Can you work these out from the model? Positions are in its coordinate system, mm. Round coordinates to 2 decimals unless told otherwise and drop trailing zeros. Loops run counter-clockwise (first coordinate to the right, second up) from the corner with the lowest first, then second, coordinate; pieces in that order, holes last.
from build123d import *

# Parameters (mm, degrees)
SKETCH_1_W               = 10.16
SKETCH_1_H               = 5.08
EXTRUDE_1_DEPTH          = 8
SKETCH_2_W               = 0.6
SKETCH_2_H               = 0.6
CUT_EXTRUDE_1_DEPTH      = 10.811116144
CHAMFER_1_SIZE           = 0.5
CHAMFER_2_SIZE           = 0.5
FILLET_1_R               = 0.05
SKETCH_4_W               = 0.6
SKETCH_4_H               = 0.25
EXTRUDE_3_DEPTH          = 1
PATTERN_LINEAR_2_COUNT   = 4
PATTERN_LINEAR_2_PITCH   = 2.54
MIRROR_1_COPY_1_SKETCH_W = 0.6
MIRROR_1_COPY_1_SKETCH_H = 0.25
MIRROR_1_COPY_1_DEPTH    = 1
MIRROR_1_COPY_2_SKETCH_W = 0.6
MIRROR_1_COPY_2_SKETCH_H = 0.25
MIRROR_1_COPY_2_DEPTH    = 1
MIRROR_1_COPY_3_SKETCH_W = 0.6
MIRROR_1_COPY_3_SKETCH_H = 0.25
MIRROR_1_COPY_3_DEPTH    = 1


with BuildPart() as part:
    # 草图1 → 凸台-拉伸1 (new body)
    with BuildSketch(Plane.XY):
        Rectangle(SKETCH_1_W, SKETCH_1_H)
    extrude(amount=EXTRUDE_1_DEPTH)

    # 草图2 → 切除-拉伸1 (cut, through all)
    with BuildSketch(Plane.XY.offset(8)):
        with Locations((1.27, 1.27)):
            Rectangle(SKETCH_2_W, SKETCH_2_H)
        with Locations((-1.27, 1.27)):
            Rectangle(SKETCH_2_W, SKETCH_2_H)
        with Locations((3.81, 1.27)):
            Rectangle(SKETCH_2_W, SKETCH_2_H)
        with Locations((-1.27, -1.27)):
            Rectangle(SKETCH_2_W, SKETCH_2_H)
        with Locations((1.27, -1.27)):
            Rectangle(SKETCH_2_W, SKETCH_2_H)
        with Locations((3.81, -1.27)):
            Rectangle(SKETCH_2_W, SKETCH_2_H)
        with Locations((-3.81, -1.27)):
            Rectangle(SKETCH_2_W, SKETCH_2_H)
        with Locations((-3.81, 1.27)):
            Rectangle(SKETCH_2_W, SKETCH_2_H)
    extrude(amount=-CUT_EXTRUDE_1_DEPTH, mode=Mode.SUBTRACT)

    # 倒角1
    chamfer_1_edges = [part.edges().sort_by_distance(p)[0] for p in [
        (-3.81, 1.57, 0),
        (-3.51, 1.27, 0),
        (-3.81, 0.97, 0),
        (-4.11, 1.27, 0),
        (-0.97, 1.27, 0),
        (-1.27, 0.97, 0),
        (-1.57, 1.27, 0),
        (-1.27, 1.57, 0),
        (1.57, 1.27, 0),
        (1.27, 0.97, 0),
        (0.97, 1.27, 0),
        (1.27, 1.57, 0),
        (-3.81, -0.97, 0),
        (-3.51, -1.27, 0),
        (-3.81, -1.57, 0),
        (-4.11, -1.27, 0),
        (4.11, 1.27, 0),
        (3.81, 0.97, 0),
        (3.51, 1.27, 0),
        (3.81, 1.57, 0),
        (-0.97, -1.27, 0),
        (-1.27, -1.57, 0),
        (-1.57, -1.27, 0),
        (-1.27, -0.97, 0),
        (1.57, -1.27, 0),
        (1.27, -1.57, 0),
        (0.97, -1.27, 0),
        (1.27, -0.97, 0),
        (4.11, -1.27, 0),
        (3.81, -1.57, 0),
        (3.51, -1.27, 0),
        (3.81, -0.97, 0),
        (4.11, -1.27, 8),
        (3.81, -0.97, 8),
        (3.51, -1.27, 8),
        (3.81, -1.57, 8),
    ]]
    chamfer(chamfer_1_edges, length=CHAMFER_1_SIZE)

    # 倒角2
    chamfer_2_edges = [part.edges().sort_by_distance(p)[0] for p in [
        (-3.81, 1.57, 8),
        (-4.11, 1.27, 8),
        (-3.81, 0.97, 8),
        (-3.51, 1.27, 8),
        (-0.97, 1.27, 8),
        (-1.27, 1.57, 8),
        (-1.57, 1.27, 8),
        (-1.27, 0.97, 8),
        (1.57, 1.27, 8),
        (1.27, 1.57, 8),
        (0.97, 1.27, 8),
        (1.27, 0.97, 8),
        (-3.81, -0.97, 8),
        (-4.11, -1.27, 8),
        (-3.81, -1.57, 8),
        (-3.51, -1.27, 8),
        (4.11, 1.27, 8),
        (3.81, 1.57, 8),
        (3.51, 1.27, 8),
        (3.81, 0.97, 8),
        (-0.97, -1.27, 8),
        (-1.27, -0.97, 8),
        (-1.57, -1.27, 8),
        (-1.27, -1.57, 8),
        (1.57, -1.27, 8),
        (1.27, -0.97, 8),
        (0.97, -1.27, 8),
        (1.27, -1.57, 8),
    ]]
    chamfer(chamfer_2_edges, length=CHAMFER_2_SIZE)

    # 圆角1
    fillet_1_edges = [part.edges().sort_by_distance(p)[0] for p in [
        (-5.08, 0, 8),
        (0, -2.54, 8),
        (5.08, 0, 8),
        (0, 2.54, 8),
        (5.08, -2.54, 4),
        (-5.08, -2.54, 4),
        (-5.08, 2.54, 4),
        (5.08, 2.54, 4),
    ]]
    fillet(fillet_1_edges, radius=FILLET_1_R)

    # 草图4 → 凸台-拉伸3 (add)
    with BuildSketch(Plane(origin=(0, 2.54, 0), x_dir=(1, 0, 0), z_dir=(0, 1, 0))):
        with Locations((-3.81, -0.125)):
            Rectangle(SKETCH_4_W, SKETCH_4_H)
    extrude_3 = extrude(amount=EXTRUDE_3_DEPTH)

    # 阵列(线性)2: 凸台-拉伸3 ×4
    with Locations(*[(i * PATTERN_LINEAR_2_PITCH, 0, 0) for i in range(1, PATTERN_LINEAR_2_COUNT)]):
        add(extrude_3)

    # 镜向1: 凸台-拉伸3 across plane
    add(extrude_3.mirror(Plane.ZX))

    # 镜向1 copy 1 sketch → 镜向1 copy 1 (add)
    with BuildSketch(Plane(origin=(2.54, -2.54, 0), x_dir=(1, 0, 0), z_dir=(0, -1, 0))):
        with Locations((-3.81, 0.125)):
            Rectangle(MIRROR_1_COPY_1_SKETCH_W, MIRROR_1_COPY_1_SKETCH_H)
    extrude(amount=MIRROR_1_COPY_1_DEPTH)

    # 镜向1 copy 2 sketch → 镜向1 copy 2 (add)
    with BuildSketch(Plane(origin=(5.08, -2.54, 0), x_dir=(1, 0, 0), z_dir=(0, -1, 0))):
        with Locations((-3.81, 0.125)):
            Rectangle(MIRROR_1_COPY_2_SKETCH_W, MIRROR_1_COPY_2_SKETCH_H)
    extrude(amount=MIRROR_1_COPY_2_DEPTH)

    # 镜向1 copy 3 sketch → 镜向1 copy 3 (add)
    with BuildSketch(Plane(origin=(7.62, -2.54, 0), x_dir=(1, 0, 0), z_dir=(0, -1, 0))):
        with Locations((-3.81, 0.125)):
            Rectangle(MIRROR_1_COPY_3_SKETCH_W, MIRROR_1_COPY_3_SKETCH_H)
    extrude(amount=MIRROR_1_COPY_3_DEPTH)


solid = part.part
(1) If I drill on line 1 (X direction, y = 1.25, z = 4.5); line 2 (Y direction, x = 0, z = 6.5); line 3 (Z direction, x = 0.75, y = -1), over which ranges is the centre line in solid material (lowest first)?
Worked answers:
line 1: x = -5.08 to -4.11, -3.51 to -1.57, -0.97 to 0.97, 1.57 to 3.51, 4.11 to 5.08
line 2: y = -2.54 to 2.54
line 3: z = 0.28 to 7.72
(2) Will these pins go through, and if not, where does the flat tip stop? P1, Ø1, axis at x = 0.5, z = 7, coming from the +Y side; P2, Ø0.5, axis at x = -1, z = 4, coming from the -Y side.
Worked answers:
P1: stops at y = 2.54
P2: stops at y = -2.54
(3) If we section it at C-C, the plane z = 1: State how many separate pieces and enclosed holes the cut face has, then the cut area to 3 significant figures.
Worked answers:
separate pieces: 1
enclosed holes: 8
area: 48.7 mm2
(4) If we section it at B-B, the plane x = -2.75: List the corners of the cut face in (y, z) for me, then the cut area to 3 significant figures.
Worked answers:
outline: (-2.54, 0) - (2.54, 0) - (2.54, 7.95) arc R0.05 ccw to (2.49, 8) - (-2.49, 8) arc R0.05 ccw to (-2.54, 7.95) - close
area: 40.6 mm2
(5) If we section it at A-A, the plane y = -3: List the corners of the cut face in (x, z) for me, then the cut area to 3 significant figures.
Worked answers:
outline: (-4.11, 0) - (-3.51, 0) - (-3.51, 0.25) - (-4.11, 0.25) - close; (-1.57, 0) - (-0.97, 0) - (-0.97, 0.25) - (-1.57, 0.25) - close; (0.97, 0) - (1.57, 0) - (1.57, 0.25) - (0.97, 0.25) - close; (3.51, 0) - (4.11, 0) - (4.11, 0.25) - (3.51, 0.25) - close
area: 0.600 mm2
